For this review, use the dimensioned drawing (mm, ordinates from the lowest corner) and the shaded views. Coordinates: 2 decimals unless noted, no trailing zeros. Loops run counter-clockwise (first coordinate to the right, second up) from the corner with the lowest first, then second, coordinate; pieces in that order, holes last. Notation, with made-up numbers: M 18,-36.75 L 42,-36.75 A8 ccw 42,-28.75 Z; hole C 85,63 d5. An arc over 180 degrees is marked long. Write each question's results on one line, items separated by ' | '. Start each with the question number.
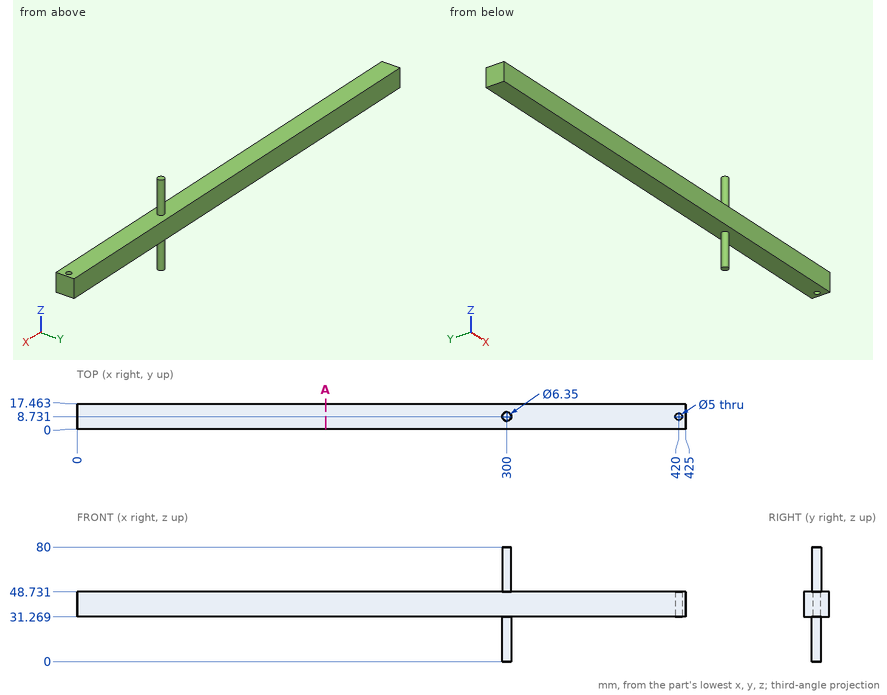
Q1. Take a section at A-A, the plane x = 173.5. Give the boundary of the cut face in (y, z).
Q2. Insertion check: P1, Ø8, axis at x = 420, y = 8.73, coming from the -Z side; P2, Ø1, axis at x = 168, y = 5.5, coming from the +Z side; P3, Ø2, axis at y = 9, z = 13, coming from the -X side (1 decimal). Each pin has a flat end and moves straight along its axis. Give the tip position at first contact, or say it passes through.
Q3. To check wall thickness, follow line 1 along Y through (x, z) = (420, 44); line 2 along Z through (x, y) = (364.5, 9.5); line 3 along X through (y, z) = (9.25, 74). State the ranges of each line that lie inside material, in increasing order.
Results:
1) outline: M 0,31.27 L 17.46,31.27 L 17.46,48.73 L 0,48.73 Z
2) P1: z = 31.27 | P2: z = 48.73 | P3: x = 296.8
3) line 1: 0 to 6.23, 11.23 to 17.46 | line 2: 31.27 to 48.73 | line 3: 296.87 to 303.13
